Source: CAD feature listing. Evaluate the final solid. Frame: model axes, mm. A direction names the side the tool comes from. Coordinates: 2 decimals unless noted, no trailing zeros. Order: outer loops, then holes, each group sorted by start corner. A loop starts at its lowest first (then second) coordinate and runs counter-clockwise, first axis right, second up.
```python
from build123d import *

# Parameters (mm, degrees)
SKETCH_1_W          = 30
SKETCH_1_H          = 300
SKETCH_1_R          = 4
EXTRUDE_1_DEPTH     = 3
EXTRUDE_2_DEPTH     = 10
EXTRUDE_3_DEPTH     = 10
EXTRUDE_4_DEPTH     = 10
SKETCH_13_R         = 1.5
CUT_EXTRUDE_1_DEPTH = 20
FILLET_1_R          = 10


with BuildPart() as part:
    # 草图1 → 凸台-拉伸1 (new body)
    # profile 1 of 2: a face of its own
    with BuildSketch(Plane.XY):
        with Locations((-15, 150)):
            Rectangle(SKETCH_1_W, SKETCH_1_H)
        with Locations((-15, 69.99339056)):
            Circle(SKETCH_1_R, mode=Mode.SUBTRACT)
        with Locations((-15, 249.99339056)):
            Circle(SKETCH_1_R, mode=Mode.SUBTRACT)
    # profile 2 of 2: a face of its own
    with BuildSketch(Plane.XY):
        with Locations((-15, -150)):
            Rectangle(SKETCH_1_W, SKETCH_1_H)
        with Locations((-15, -290.00660944)):
            Circle(SKETCH_1_R, mode=Mode.SUBTRACT)
        with Locations((-15, -110.00660944)):
            Circle(SKETCH_1_R, mode=Mode.SUBTRACT)
    extrude(amount=EXTRUDE_1_DEPTH)

    # 草图10 → 凸台-拉伸2 (add, symmetric)
    with BuildSketch(Plane(origin=(0, -20.00660944, 0), x_dir=(1, 0, 0), z_dir=(0, 1, 0))):
        with BuildLine():
            Line((-30, 0), (4.616994756, 0))
            ThreePointArc((4.616994756, 0), (15.2, -8), (25.783005244, 0))
            Line((25.783005244, 0), (35.2, 0))
            Line((35.2, 0), (35.2, 3))
            Line((35.2, 3), (25.2, 3))
            ThreePointArc((25.2, 3), (15.2, -7), (5.2, 3))
            Line((5.2, 3), (-30, 3))
            Line((-30, 3), (-30, 0))
        make_face()
    extrude(amount=EXTRUDE_2_DEPTH, both=True)

    # 草图11 → 凸台-拉伸3 (add, symmetric)
    with BuildSketch(Plane(origin=(0, 159.99339056, 0), x_dir=(1, 0, 0), z_dir=(0, 1, 0))):
        with BuildLine():
            Line((-30, 0), (4.616994756, 0))
            ThreePointArc((4.616994756, 0), (15.2, -8), (25.783005244, 0))
            Line((25.783005244, 0), (35.2, 0))
            Line((35.2, 0), (35.2, 3))
            Line((35.2, 3), (25.2, 3))
            ThreePointArc((25.2, 3), (15.2, -7), (5.2, 3))
            Line((5.2, 3), (-30, 3))
            Line((-30, 3), (-30, 0))
        make_face()
    extrude(amount=EXTRUDE_3_DEPTH, both=True)

    # 草图12 → 凸台-拉伸4 (add, symmetric)
    with BuildSketch(Plane(origin=(0, -170.00660944, 0), x_dir=(1, 0, 0), z_dir=(0, 1, 0))):
        with BuildLine():
            Line((-30, 0), (4.616994756, 0))
            ThreePointArc((4.616994756, 0), (15.2, -8), (25.783005244, 0))
            Line((25.783005244, 0), (35.2, 0))
            Line((35.2, 0), (35.2, 3))
            Line((35.2, 3), (25.2, 3))
            ThreePointArc((25.2, 3), (15.2, -7), (5.2, 3))
            Line((5.2, 3), (-30, 3))
            Line((-30, 3), (-30, 0))
        make_face()
    extrude(amount=EXTRUDE_4_DEPTH, both=True)

    # 草图13 → 切除-拉伸1 (cut)
    with BuildSketch(Plane.XY.offset(3)):
        with Locations((30.491502622, 164.99339056)):
            Circle(SKETCH_13_R)
        with Locations((30.491502622, 154.99339056)):
            Circle(SKETCH_13_R)
        with Locations((-10.5, 154.99339056)):
            Circle(SKETCH_13_R)
        with Locations((-10.5, 164.99339056)):
            Circle(SKETCH_13_R)
        with Locations((30.491502622, -15.00660944)):
            Circle(SKETCH_13_R)
        with Locations((30.491502622, -25.00660944)):
            Circle(SKETCH_13_R)
        with Locations((-10.5, -25.00660944)):
            Circle(SKETCH_13_R)
        with Locations((-10.5, -15.00660944)):
            Circle(SKETCH_13_R)
        with Locations((30.491502622, -165.00660944)):
            Circle(SKETCH_13_R)
        with Locations((30.491502622, -175.00660944)):
            Circle(SKETCH_13_R)
        with Locations((-10.5, -175.00660944)):
            Circle(SKETCH_13_R)
        with Locations((-10.5, -165.00660944)):
            Circle(SKETCH_13_R)
    extrude(amount=-CUT_EXTRUDE_1_DEPTH, mode=Mode.SUBTRACT)

    # 圆角1
    # the kernel refuses this fillet: 10 mm, written as the material it adds along each edge
    with BuildSketch(Plane(origin=(-30, -160.00660944, 0), x_dir=(0, 1, 0), z_dir=(1, 0, 0)), Plane(origin=(-30, -10.00660944, 0), x_dir=(0, 1, 0), z_dir=(1, 0, 0)), Plane(origin=(-30, 169.99339056, 0), x_dir=(0, 1, 0), z_dir=(1, 0, 0))) as fillet_1_piece_1:
        with BuildLine():
            CenterArc((7.141428429, -10), FILLET_1_R, 90, 45.572995999)
            Line((0, -3), (0, 0))
            Line((0, 0), (7.141428429, 0))
        make_face()
    extrude(amount=30)
    with BuildSketch(Plane(origin=(-30, -180.00660944, 0), x_dir=(0, -1, 0), z_dir=(1, 0, 0)), Plane(origin=(-30, -30.00660944, 0), x_dir=(0, -1, 0), z_dir=(1, 0, 0)), Plane(origin=(-30, 149.99339056, 0), x_dir=(0, -1, 0), z_dir=(1, 0, 0))) as fillet_1_piece_2:
        with BuildLine():
            CenterArc((7.141428429, 10), FILLET_1_R, 224.427004001, 45.572995999)
            Line((0, 3), (0, 0))
            Line((0, 0), (7.141428429, 0))
        make_face()
    extrude(amount=30)


solid = part.part
```
1. Section query C-C on y = 260.5. Return loops of the section in (x, z).
Findings:
outline: (-30, 0) - (0, 0) - (0, 3) - (-30, 3) - close
2. Draft query along X for faces 6 (the face through (15, 160, 7)), 7 (the face through (30, -170, 0)). Return one class per face: released by +X, released by -X, zero draft, split by the parting line, or undercut.
Findings:
face 6: undercut
face 7: zero draft
3. Section query B-B on z = 4.75. Return loops of the section in (x, y), plus the area to 3 significant figures.
Findings:
outline: (7.39, -180.01) - (8.88, -180.01) - (8.88, -160.01) - (7.39, -160.01) - close; (7.39, -30.01) - (8.88, -30.01) - (8.88, -10.01) - (7.39, -10.01) - close; (7.39, 149.99) - (8.88, 149.99) - (8.88, 169.99) - (7.39, 169.99) - close; (21.52, -180.01) - (23.01, -180.01) - (23.01, -160.01) - (21.52, -160.01) - close; (21.52, -30.01) - (23.01, -30.01) - (23.01, -10.01) - (21.52, -10.01) - close; (21.52, 149.99) - (23.01, 149.99) - (23.01, 169.99) - (21.52, 169.99) - close
area: 178 mm2
4. Pin query (flat end, axial travel): P1, Ø3, axis at x = 30, y = -173.5, coming from the +Z side; P2, Ø10.5, axis at x = 30.5, y = 159.5, coming from the +Z side; P3, Ø1, axis at y = 115.5, z = 0.5, coming from the +X side; P4, Ø1.8, axis at x = -10.5, y = 164.99, coming from the +Z side. Return the tip coordinate at first contact, or that it passes through.
Findings:
P1: stops at z = 0
P2: stops at z = 1.47
P3: stops at x = 0
P4: passes through
5. Section query A-A on x = 15.2. Return loops of the section in (y, z), plus the area to 3 significant figures.
Findings:
outline: (-180.01, 7) - (-160.01, 7) - (-160.01, 8) - (-180.01, 8) - close; (-30.01, 7) - (-10.01, 7) - (-10.01, 8) - (-30.01, 8) - close; (149.99, 7) - (169.99, 7) - (169.99, 8) - (149.99, 8) - close
area: 60.0 mm2
6. Access query for faces 1 (the face through (23, -160.007, 4)), 2 (the face through (-15, 239, 0)), 3 (the face through (23, 169.993, 4)), 4 (the face through (-15, -243, 0)), 5 (the face through (23, -180.007, 4)). Directions: +Z, -Z, +X, -X, +Y, -Y. A direction counts if a zero-diameter tool reaches every point of the face in a straight line with its end or side. Return the directions, or none.
Findings:
face 1: +Z, -Z, +X
face 2: -Z, +X, -X, +Y
face 3: +Z, -Z, +X, +Y
face 4: -Z, +X, -X, -Y
face 5: +Z, -Z, +X, -Y
7. Ray query, line 1 (Y direction, x = -15, z = 1.3); line 2 (Y direction, x = 8.5, z = 5); line 3 (Z direction, x = 26.5, y = -26.5). Return the intervals inside material, ascending.
Findings:
line 1: y = -300 to -294.01, -286.01 to -114.01, -106.01 to 65.99, 73.99 to 245.99, 253.99 to 300
line 2: y = -180.01 to -160.01, -30.01 to -10.01, 149.99 to 169.99
line 3: z = -3 to 0
